The model under review builds one solid part; all positions refer to its coordinate system, in mm. A direction names the side the tool comes from. Give positions to 0.01 mm unless a question says otherwise; leave off trailing zeros. Loops run counter-clockwise (first coordinate to the right, second up) from the corner with the lowest first, then second, coordinate; pieces in that order, holes last. Notation, with made-up numbers: (50.25, -21.5) - (81.25, -21.5) arc R23 cw to (81.25, -10.5) - close; hole circle Ø11 at (62.25, 47). An arc over 180 degrees is marked (long way). Return JSON: item names as keys, results as strings. Group by question number.
```python
from build123d import *

# Parameters (mm, degrees)
SKIZZE1_W                       = 88.6
SKIZZE1_H                       = 59.6
AUFSATZ_LINEAR_AUSTRAGEN1_DEPTH = 1.8
SCHNITT_LINEAR_AUSTRAGEN1_DEPTH = 54.420688876
FASE1_SIZE                      = 0.5
AUFSATZ_LINEAR_AUSTRAGEN2_DEPTH = 5
AUFSATZ_LINEAR_AUSTRAGEN3_DEPTH = 5
VERRUNDUNG1_R                   = 0.8
SKIZZE5_W                       = 2.5
SKIZZE5_H                       = 11.6
SCHNITT_LINEAR_AUSTRAGEN2_DEPTH = 57.896671713
VERRUNDUNG2_R                   = 0.8


with BuildPart() as part:
    # Skizze1 → Aufsatz-Linear austragen1 (new body)
    with BuildSketch(Plane(origin=(0, 0, 0), x_dir=(1, 0, 0), z_dir=(0, 1, 0))):
        Rectangle(SKIZZE1_W, SKIZZE1_H)
    extrude(amount=AUFSATZ_LINEAR_AUSTRAGEN1_DEPTH)

    # Skizze2 → Schnitt-Linear austragen1 (cut, through all)
    with BuildSketch(Plane(origin=(0, 1.8, 0), x_dir=(1, 0, 0), z_dir=(0, 1, 0))):
        with BuildLine():
            Line((-44.3, -29.8), (-41.5, -29.8))
            ThreePointArc((-41.5, -29.8), (-43.479898987, -28.979898987), (-44.3, -27))
            Line((-44.3, -27), (-44.3, -29.8))
        make_face()
        with BuildLine():
            Line((41.5, -29.8), (44.3, -29.8))
            Line((44.3, -29.8), (44.3, -27))
            ThreePointArc((44.3, -27), (43.479898987, -28.979898987), (41.5, -29.8))
        make_face()
        with BuildLine():
            ThreePointArc((41.5, 29.8), (43.479898987, 28.979898987), (44.3, 27))
            Line((44.3, 27), (44.3, 29.8))
            Line((44.3, 29.8), (41.5, 29.8))
        make_face()
        with BuildLine():
            ThreePointArc((-44.3, 27), (-43.479898987, 28.979898987), (-41.5, 29.8))
            Line((-41.5, 29.8), (-44.3, 29.8))
            Line((-44.3, 29.8), (-44.3, 27))
        make_face()
    extrude(amount=-SCHNITT_LINEAR_AUSTRAGEN1_DEPTH, mode=Mode.SUBTRACT)

    # Fase1
    fase1_edges = [part.edges().sort_by_distance(p)[0] for p in [
        (44.3, 1.8, 0),
        (0, 1.8, -29.8),
        (-44.3, 1.8, 0),
        (0, 1.8, 29.8),
        (-43.479898987, 1.8, -28.979898987),
        (43.479898987, 1.8, -28.979898987),
        (43.479898987, 1.8, 28.979898987),
        (-43.479898987, 1.8, 28.979898987),
    ]]
    chamfer(fase1_edges, length=FASE1_SIZE)

    # Skizze3 → Aufsatz-Linear austragen2 (add, symmetric)
    with BuildSketch(Plane.XY):
        with BuildLine():
            Line((44.5, 0), (40.5, 0))
            ThreePointArc((40.5, 0), (41.207106781, -0.292893219), (41.5, -1))
            ThreePointArc((41.5, -1), (41.792893219, -1.707106781), (42.5, -2))
            Line((42.5, -2), (44.5, -2))
            ThreePointArc((44.5, -2), (45.5, -1), (44.5, 0))
        make_face()
    extrude(amount=AUFSATZ_LINEAR_AUSTRAGEN2_DEPTH, both=True)

    # Skizze4 → Aufsatz-Linear austragen3 (add, symmetric)
    with BuildSketch(Plane.XY):
        with BuildLine():
            Line((-44.3, 0), (-44.3, -8))
            Line((-44.3, -8), (-47, -8))
            Line((-47, -8), (-47, -9.5))
            Line((-47, -9.5), (-45, -11.5))
            ThreePointArc((-45, -11.5), (-43.963143632, -11.801551092), (-43.239596788, -11))
            Line((-43.239596788, -11), (-41.3, 0))
            Line((-41.3, 0), (-44.3, 0))
        make_face()
    extrude(amount=AUFSATZ_LINEAR_AUSTRAGEN3_DEPTH, both=True)

    # Verrundung1
    verrundung1_edges = [part.edges().sort_by_distance(p)[0] for p in [
        (-42.8, 0, -5),
        (-42.8, 0, 5),
    ]]
    fillet(verrundung1_edges, radius=VERRUNDUNG1_R)

    # Skizze5 → Schnitt-Linear austragen2 (cut, through all)
    with BuildSketch(Plane.XZ):
        with Locations((-40.05, 0)):
            Rectangle(SKIZZE5_W, SKIZZE5_H)
    extrude(amount=-SCHNITT_LINEAR_AUSTRAGEN2_DEPTH, mode=Mode.SUBTRACT)

    # Verrundung2
    # the kernel refuses this fillet: 0.8 mm, written as the material it adds along each edge
    with BuildSketch(Plane(origin=(-41.3, 0, -5.8), x_dir=(1, 0, 0), z_dir=(0, 1, 0))) as verrundung2_piece_1:
        with BuildLine():
            CenterArc((VERRUNDUNG2_R, -VERRUNDUNG2_R), VERRUNDUNG2_R, 90, 90)
            Line((0, -VERRUNDUNG2_R), (0, 0))
            Line((0, 0), (VERRUNDUNG2_R, 0))
        make_face()
    extrude(amount=1.8)
    with BuildSketch(Plane(origin=(-41.3, 0, 5.8), x_dir=(1, 0, 0), z_dir=(0, 1, 0)), Plane(origin=(-38.8, 0, 5.8), x_dir=(0, 0, -1), z_dir=(0, 1, 0)), Plane(origin=(-38.8, 0, -5.8), x_dir=(-1, 0, 0), z_dir=(0, 1, 0))) as verrundung2_piece_2:
        with BuildLine():
            CenterArc((VERRUNDUNG2_R, VERRUNDUNG2_R), VERRUNDUNG2_R, 180, 90)
            Line((0, VERRUNDUNG2_R), (0, 0))
            Line((0, 0), (VERRUNDUNG2_R, 0))
        make_face()
    extrude(amount=1.8)


solid = part.part
```
1) We need section C-C, the plane y = -6. Write out the cut boundary in (x, z).
2) Tool access review of faces 4 (the face through (-46, -8, 0)), 5 (the face through (43, -2, 0)), 6 (the face through (-44, -6, 5)), 7 (the face through (-42.283, -5.577, 0.081)): name each direction out of +Z, -Z, +X, -X, +Y, -Y from which nothing blocks a thin tool from reaching the whole face with its end or side.
3) For pin 1 Ø0.8 at (x, z) = (-46, 1) entering from +Y; pin 2 Ø2 at (y, z) = (1, -1) entering from -X; pin 3 Ø1 at (y, z) = (1, 12.5) entering from +X; pin 4 Ø4.5 at (y, z) = (-3, 11) entering from -X, all flat-tipped, find the tip position at first contact; note any pin that passes through.
4) Draft analysis for pull direction X (two halves, no side actions). For faces 1 (the face through (45.5, -1, 0.1)), 2 (the face through (-38.8, 1, 0)), 3 (the face through (-44.3, -2, 0)), state which applies: +X half, -X half, draft (parallel to the pull), parting line (faces both ways), or undercut.
5) We need section B-B, the plane z = -16.5. Write out the cut boundary in (x, y), plus the area to 3 significant figures.
6) To check wall thickness, follow line 1 (Y direction, x = 12.5, z = -2.5); line 2 (X direction, y = -5, z = 2); line 3 (X direction, y = -11, z = 0.5). State the ranges of each line that lie inside material, in increasing order.
7) We need section A-A, the plane x = -12. Write out the cut boundary in (y, z).
Findings:
{
 "1": {"outline": "(-44.3, -5) - (-42.36, -5) - (-42.36, 5) - (-44.3, 5) - close"},
 "2": {"face 4": "+Z, -Z, -X, +Y", "face 5": "+Z, -Z, +X, -Y", "face 6": "+Z, +X, -X, -Y", "face 7": "+Z, -Z, -Y"},
 "3": {"pin 1": "stops at y = -8", "pin 2": "stops at x = -44.3", "pin 3": "stops at x = 44.3", "pin 4": "passes through"},
 "4": {"face 1": "+X half", "face 2": "undercut", "face 3": "-X half"},
 "5": {"outline": "(-44.3, 0) - (44.3, 0) - (44.3, 1.3) - (43.8, 1.8) - (-43.8, 1.8) - (-44.3, 1.3) - close", "area": "159 mm^2"},
 "6": {"line 1": "y = 0 to 1.8", "line 2": "x = -44.3 to -42.18", "line 3": "x = -45.5 to -43.24"},
 "7": {"outline": "(0, -29.8) - (1.3, -29.8) - (1.8, -29.3) - (1.8, 29.3) - (1.3, 29.8) - (0, 29.8) - close"}
}
